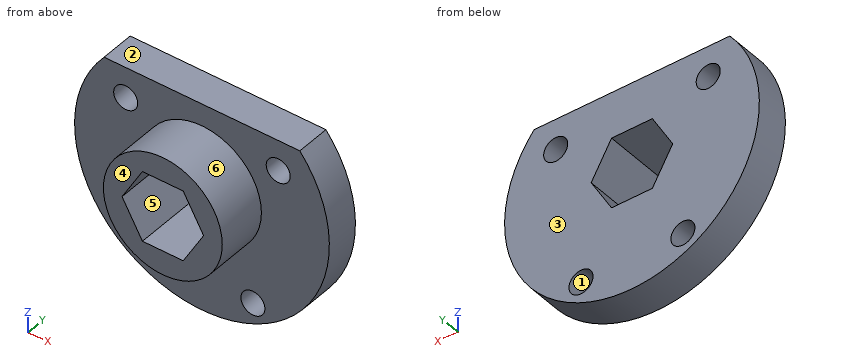
from build123d import *

# Parameters (mm, degrees)
F1_DEPTH = 6.35
F3_D     = 4.4958
F4_R     = 11.1125
F5_DEPTH = 9.525
F7_DEPTH = 15.876


with BuildPart() as f1:
    # F0 (on Front) → F1 (new body)
    with BuildSketch(Plane.XZ):
        with BuildLine():
            Line((18.2969275085, 15.24), (-18.2969275085, 15.24))
            ThreePointArc((-18.2969275085, 15.24), (0, -23.8125), (18.2969275085, 15.24))
        make_face()
    extrude(amount=F1_DEPTH)

    # F3 (through all)
    with Locations(Plane.XZ.offset(6.35)):
        with Locations((-14.2575098316, 9.525), (14.2575098316, 9.525), (9.525, -17.8901402442), (-9.525, -17.8901402442)):
            Hole(F3_D / 2)

    # F4 (on face) → F5 (join)
    with BuildSketch(Plane.XZ.offset(6.35)):
        Circle(F4_R)
    extrude(amount=F5_DEPTH)

    # F6 (on face) → F7 (cut, through all)
    with BuildSketch(Plane.XZ.offset(15.875)):
        Polygon((3.8128211777, -6.604), (7.6256423555, 0), (3.8128211777, 6.604), (-3.8128211777, 6.604), (-7.6256423555, 0), (-3.8128211777, -6.604), align=None)
    extrude(amount=-F7_DEPTH, mode=Mode.SUBTRACT)


solid = f1.part
Can you work these out from the model? Positions are in its coordinate system, mm. Face numbers are marked on the shaded views. A direction names the side the tool comes from. Give positions to 0.01 mm unless a question says otherwise; leave off trailing zeros. Order: outer loops, then holes, each group sorted by start corner. A loop starts at its lowest first (then second) coordinate and runs counter-clockwise, first axis right, second up. Notation, with made-up numbers: M 41.5,-19.75 L 50.5,-19.75 A28 cw 50.5,4.25 Z; hole C -20,-15.5 d11. An arc over 180 degrees is marked long. Use a Markdown table: item, result. Add a question column.
Item 1: Suppose I cut it at C-C (z = -1.5). List the corners of the cut face in (x, y) for me (3 decimals), then the cut area to 3 significant figures.
Item 2: Will these pins go through, and if not, where does the flat tip stop? pin 1 (4 mm diameter, centred on x = -14.26, z = 9.52, fed in from -Y); pin 2 (7 mm diameter, centred on x = -9.52, z = -17.89, fed in from -Y); pin 3 (2 mm diameter, centred on y = -9.5, z = -11, fed in from -X); pin 4 (5 mm diameter, centred on x = -12.5, y = -3, fed in from -Z).
Item 3: We'd pull the mould along Z, two halves only. Please class the marked faces 1, 2 and 3: +Z half, -Z half, draft (parallel to the pull), parting line (faces both ways), or undercut.
Item 4: Suppose I cut it at B-B (y = -11.75). List the corners of the cut face in (x, z) for me (1 decimal), then the cut area to 3 significant figures.
Item 5: Suppose I cut it at D-D (y = -2.75). List the corners of the cut face in (x, z) for me (1 decimal).
Item 6: If I drill on L1, parallel to X at y = -5.25, z = 10.5; L2, parallel to X at y = -4.5, z = 0; L3, parallel to Z at x = 5, y = -8, over which ranges is the centre line in solid material (lowest first)? Write a range as [from, to].
Item 7: For the marked faces 4, 5 and 6, which set-ups out of +Z, -Z, +X, -X, +Y, -Y let a thin tool reach every point of the face, with its end or its side?
Answer sheet:
| question | item | result |
|---|---|---|
| 1 | outline | M -23.765,-6.35 L -11.011,-6.35 L -11.011,-15.875 L -6.76,-15.875 L -6.76,0 L -23.765,0 Z; M 6.76,-15.875 L 11.011,-15.875 L 11.011,-6.35 L 23.765,-6.35 L 23.765,0 L 6.76,0 Z |
| 1 | area | 297 mm² |
| 2 | pin 1 | passes through |
| 2 | pin 2 | stops at y = -6.35 |
| 2 | pin 3 | stops at x = -4.85 |
| 2 | pin 4 | stops at z = -21.61 |
| 3 | face 1 | undercut |
| 3 | face 2 | +Z half |
| 3 | face 3 | draft |
| 4 | outline | C 0,0 d22.2; hole M -7.6,0 L -3.8,-6.6 L 3.8,-6.6 L 7.6,0 L 3.8,6.6 L -3.8,6.6 Z |
| 4 | area | 237 mm² |
| 5 | outline | M -18.3,15.2 A23.8 ccw long 18.3,15.2 Z; hole C -14.3,9.5 d4.5; hole C -9.5,-17.9 d4.5; hole M -7.6,0 L -3.8,-6.6 L 3.8,-6.6 L 7.6,0 L 3.8,6.6 L -3.8,6.6 Z; hole C 9.5,-17.9 d4.5; hole C 14.3,9.5 d4.5 |
| 6 | L1 | x = [-21.37, -16.28], [-12.23, 12.23], [16.28, 21.37] |
| 6 | L2 | x = [-23.81, -7.63], [7.63, 23.81] |
| 6 | L3 | z = [-9.92, -4.55], [4.55, 9.92] |
| 7 | face 4 | +Z, -Z, +X, -X, -Y |
| 7 | face 5 | +Y, -Y |
| 7 | face 6 | -Y |
